Geometry: see drawing. Coordinates: mm, zero at the bounding-box minimum. A direction names the side the tool comes from. Give positions to 0.01 mm unless a question says otherwise; leave off trailing zeros. Write each loop counter-clockwise with the first axis right and the second up, starting at its lowest first coordinate (ties: lowest second). Pieces come first, ordered by that corner, then holes. Notation, with made-up numbers: (39, 56.5) -> (52, 56.5) arc R24 ccw to (52, 73.5) -> close; hole circle Ø6 at (-7.5, 26). An arc over 180 degrees is marked (long way). Use CSV: the item, a comma, the result in double quotes. Start each with the question number.
1) Section D-D (z = 28). Output: boundary loops of the cut face in (x, y), plus the area to 3 significant figures.
2) Draft query along X for the marked faces 4, 5 and 6. Return one class per face: pulls with the +X half, pulls with the -X half, needs draft (parallel to the pull), parting line crosses it, or undercut.
3) Section C-C (x = 15). Output: boundary loops of the cut face in (y, z), plus the area to 3 significant figures.
4) Material intervals for line 1 (X direction, y = 13, z = 33); line 2 (Z direction, x = 19, y = 18.5); line 3 (Y direction, x = 12, z = 33.5), sorted ascending. Write a range as [from, to].
5) Contact query for flat-ended pins moving along their axis: P1, Ø3, axis at x = 32, z = 28.5, coming from the -Y side; P2, Ø8, axis at x = 19.5, z = 36, coming from the -Y side; P3, Ø5.5, axis at x = 18.5, y = 18.5, coming from the +Z side. Output: stop coordinate, or through.
6) Section A-A (z = 8). Output: boundary loops of the cut face in (x, y), plus the area to 3 significant figures.
7) Section B-B (y = 31.5). Output: boundary loops of the cut face in (x, z), plus the area to 3 significant figures.
8) Set-up query: the marked faces 1, 2 and 3. Return all of +Z, -Z, +X, -X, +Y, -Y with unobstructed straight access to the full face (end or side cutting, diameter ignored); none if empty.
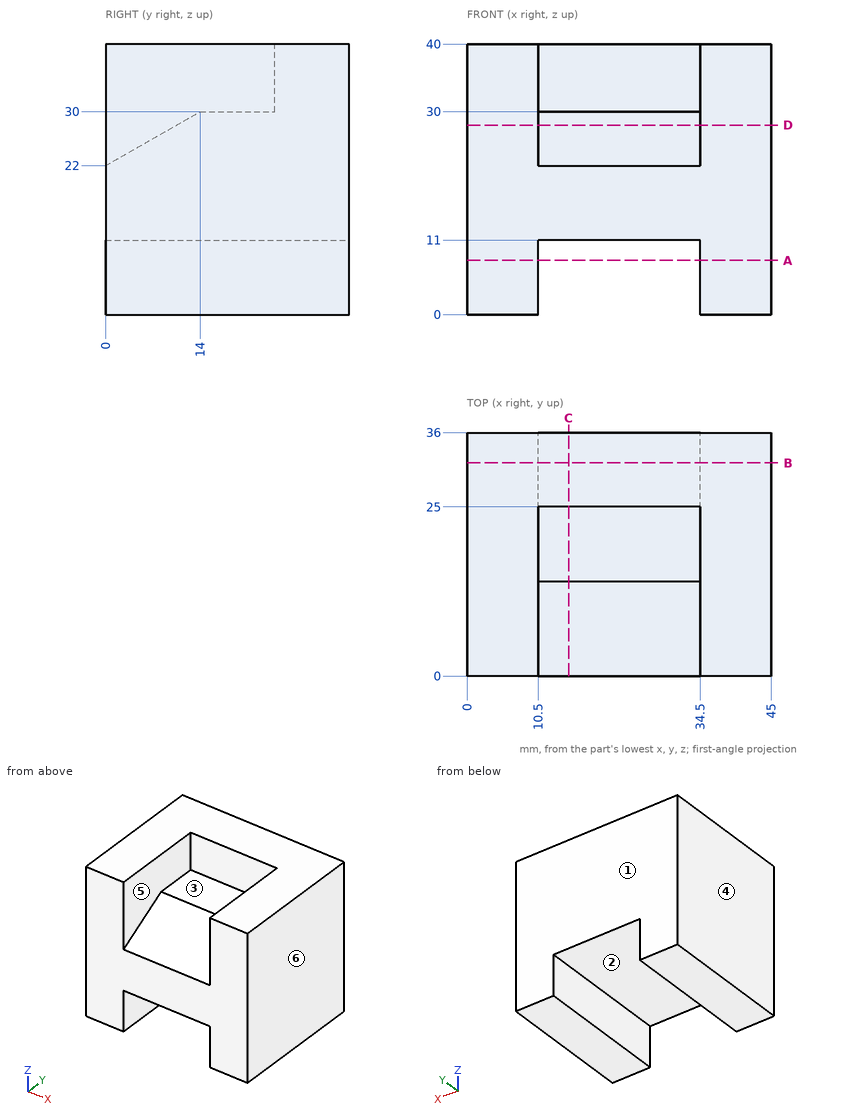
Answers follow:
1,outline,"(0, 0) -> (10.5, 0) -> (10.5, 10.5) -> (34.5, 10.5) -> (34.5, 0) -> (45, 0) -> (45, 36) -> (0, 36) -> close"
1,area,"1,370 mm^2"
2,face 4,"pulls with the -X half"
2,face 5,"undercut"
2,face 6,"pulls with the +X half"
3,outline,"(0, 11) -> (36, 11) -> (36, 40) -> (25, 40) -> (25, 30) -> (14, 30) -> (0, 22) -> close"
3,area,"738 mm^2"
4,line 1,"x = [0, 10.5], [34.5, 45]"
4,line 2,"z = [11, 30]"
4,line 3,"y = [25, 36]"
5,P1,"stops at y = 8.75"
5,P2,"stops at y = 25"
5,P3,"stops at z = 30"
6,outline,"(0, 0) -> (10.5, 0) -> (10.5, 36) -> (0, 36) -> close; (34.5, 0) -> (45, 0) -> (45, 36) -> (34.5, 36) -> close"
6,area,"756 mm^2"
7,outline,"(0, 0) -> (10.5, 0) -> (10.5, 11) -> (34.5, 11) -> (34.5, 0) -> (45, 0) -> (45, 40) -> (0, 40) -> close"
7,area,"1,540 mm^2"
8,face 1,"+Z, -Z, +X, -X, +Y"
8,face 2,"-Z, +Y, -Y"
8,face 3,"+Z, -Y"
